Job drawing, mm, ordinate dimensions from the low corner. One solid piece. A direction names the side the tool comes from. Round coordinates to 2 decimals unless told otherwise and drop trailing zeros. Order: outer loops, then holes, each group sorted by start corner. A loop starts at its lowest first (then second) coordinate and runs counter-clockwise, first axis right, second up. Notation, with made-up numbers: (83, 70) -> (140, 70) arc R13 cw to (140, 75) -> close; hole circle Ø1 at (4.25, -22). An arc over 180 degrees is marked (long way). Write item = value, one per line.
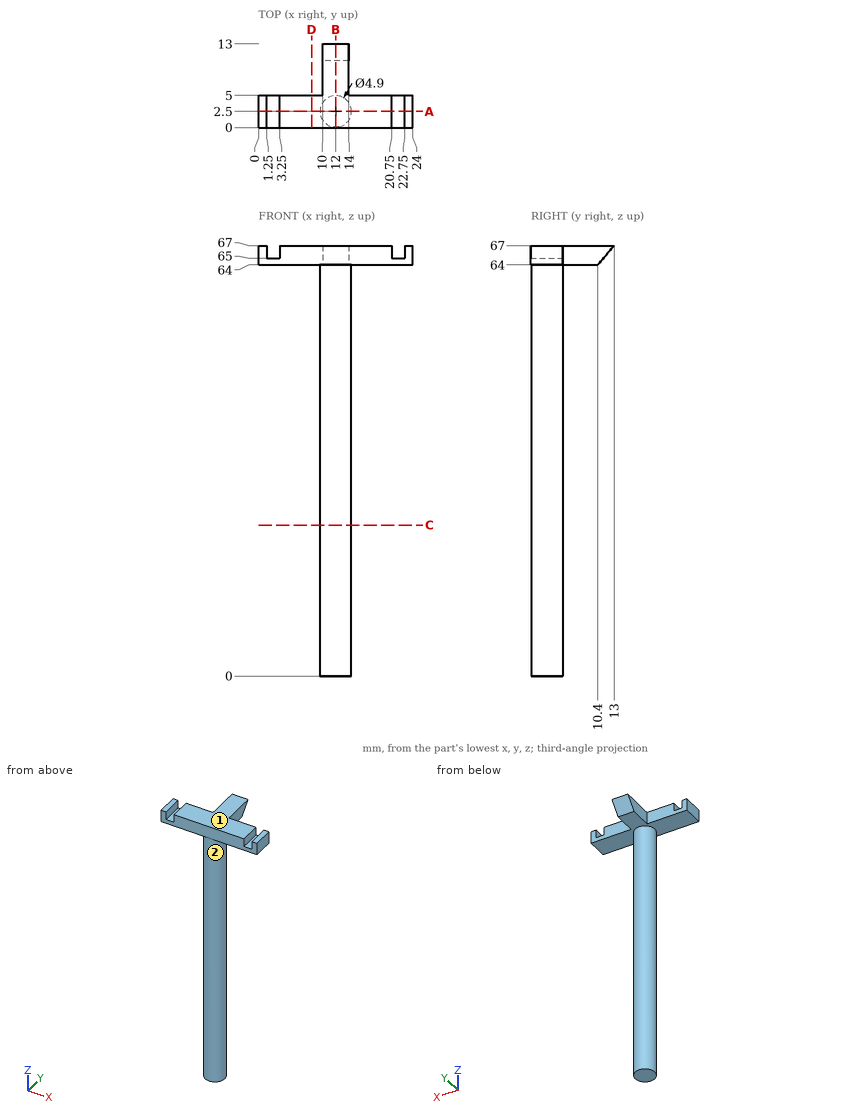
Q1. Cut at A-A, the plane y = 2.5. List the corners of the cut face in (x, z), and give its area (3 significant figures).
Check values:
outline = (0, 64) -> (9.55, 64) -> (9.55, 0) -> (14.45, 0) -> (14.45, 64) -> (24, 64) -> (24, 67) -> (22.75, 67) -> (22.75, 65) -> (20.75, 65) -> (20.75, 67) -> (3.25, 67) -> (3.25, 65) -> (1.25, 65) -> (1.25, 67) -> (0, 67) -> close
area = 378 mm²
Q2. Cut at D-D, the plane x = 8.25. List the corners of the cut face in (y, z), and give its area (3 significant figures).
Check values:
outline = (0, 64) -> (5, 64) -> (5, 67) -> (0, 67) -> close
area = 15.0 mm²
Q3. Flat gauge pins, fed straight in: pin 1 (0.6 mm diameter, centred on x = 22, y = 3, fed in from +Z); pin 2 (2.5 mm diameter, centred on y = 9.5, z = 65, fed in from -X); pin 3 (5 mm diameter, centred on x = 6, z = 52, fed in from +Y); pin 4 (12 mm diameter, centred on x = 7, z = 10, fed in from -Y). Where does each tip first touch, or does it go through?
Check values:
pin_1 = 65
pin_2 = 10
pin_3 = through
pin_4 = 0.05
Q4. Probe probe 1 along Z at (x, y) = (12.25, 6.5); probe 2 along Z at (x, y) = (21.25, 3.5); probe 3 along X at (y, z) = (2.25, 53). List the from-to ranges inside material, lowest first.
Check values:
probe_1 = 64 to 67
probe_2 = 64 to 65
probe_3 = 9.56 to 14.44
Q5. Cut at B-B, the plane x = 12. List the corners of the cut face in (y, z).
Check values:
outline = (0, 64) -> (0.05, 64) -> (0.05, 0) -> (4.95, 0) -> (4.95, 64) -> (10.4, 64) -> (13, 67) -> (0, 67) -> close
Q6. Which spindle directions (+Z, -Z, +X, -X, +Y, -Y) get a long thin tool onto all of the face, cutting with end or side? Do the marked faces 1 and 2. Say none if no direction does.
Check values:
face_1 = +Z, +X, -X, +Y, -Y
face_2 = -Z
Q7. Cut at C-C, the plane z = 23.5. List the corners of the cut face in (x, y).
Check values:
outline = circle Ø4.9 at (12, 2.5)
